Verification items for the finished model (mm, model axes). A direction names the side the tool comes from. Coordinates: 2 decimals unless noted, no trailing zeros. Order: outer loops, then holes, each group sorted by start corner. A loop starts at its lowest first (then second) coordinate and runs counter-clockwise, first axis right, second up. Notation, with made-up numbers: M 52.25,89 L 111.25,89 A33 cw 111.25,126 Z; hole C 77.5,-36.5 d1. An arc over 180 degrees is marked long. Answer as a JSON object with one key per item and string values. Group by question number.
(1) Cross-section at B-B (z = -0.7). Enter the section's corners in (x, y), plus the area to 3 significant figures.
(2) Gauge pin test, flat ends, axial feed: pin 1 Ø2 at (x, z) = (-15.5, -2.5) entering from -Y; pin 2 Ø2 at (x, z) = (-13.5, -1.5) entering from +Y; pin 3 Ø2 at (x, z) = (-7, -2.5) entering from +Y. Record the tip position at first contact, or that the pin passes through.
(3) Material ranges on line 1 (X direction, y = 3.5, z = -1.8); line 2 (X direction, y = 0.25, z = -0.95); line 3 (Y direction, x = -18.5, z = -1.65), recorded low to high.
(4) Cross-section at C-C (y = 3). Enter the section's corners in (x, z).
(5) Access from +Z, -Z, +X, -X, +Y, -Y to the whole of each face (thin tool, end or side, straight path). Record for faces 1 (the face through (-15, 3, 0)), 2 (the face through (-21.4, 5.48, -2.03)), 3 (the face through (-8.51, -0.51, -2.03)).
(6) Cross-section at A-A (x = -27.5). Enter the section's corners in (y, z).
(7) Cross-section at D-D (x = -10.5). Enter the section's corners in (y, z), plus the area to 3 significant figures.
from build123d import *

# Parameters (mm, degrees)
EXTRUDE_1_DEPTH = 4
FILLET_1_R      = 10


with BuildPart() as part:
    # ｽｹｯﾁ1 → ﾎﾞｽ - 押し出し1 (new body)
    with BuildSketch(Plane.XY):
        with BuildLine():
            Line((-0.345934077, 5), (0, 5))
            Line((0, 5), (0, 4.654065923))
            ThreePointArc((0, 4.654065923), (0.59354166, 3.648912529), (0.8, 2.5))
            ThreePointArc((0.8, 2.5), (0.59354166, 1.351087471), (0, 0.345934077))
            Line((0, 0.345934077), (0, 0))
            Line((0, 0), (-0.345934077, 0))
            ThreePointArc((-0.345934077, 0), (-2.5, -0.8), (-4.654065923, 0))
            Line((-4.654065923, 0), (-7.398979486, 0))
            ThreePointArc((-7.398979486, 0), (-1.214384811, -2.847634392), (3, 2.5))
            ThreePointArc((3, 2.5), (-1.214384811, 7.847634392), (-7.398979486, 5))
            Line((-7.398979486, 5), (-4.654065923, 5))
            ThreePointArc((-4.654065923, 5), (-2.5, 5.8), (-0.345934077, 5))
        make_face()
        with BuildLine():
            ThreePointArc((-4.654065923, 0), (-5.8, 2.5), (-4.654065923, 5))
            Line((-4.654065923, 5), (-7.398979486, 5))
            ThreePointArc((-7.398979486, 5), (-8, 2.5), (-7.398979486, 0))
            Line((-7.398979486, 0), (-4.654065923, 0))
        make_face()
        with BuildLine():
            Line((0, 0), (0, 0.345934077))
            ThreePointArc((0, 0.345934077), (-0.166547622, 0.166547622), (-0.345934077, 0))
            Line((-0.345934077, 0), (0, 0))
        make_face()
        with BuildLine():
            Line((0, 4.654065923), (0, 5))
            Line((0, 5), (-0.345934077, 5))
            ThreePointArc((-0.345934077, 5), (-0.166547622, 4.833452378), (0, 4.654065923))
        make_face()
        with BuildLine():
            ThreePointArc((-7.398979486, 0), (-8, 2.5), (-7.398979486, 5))
            Line((-7.398979486, 5), (-22.601020514, 5))
            ThreePointArc((-22.601020514, 5), (-22.152365608, 3.785615189), (-22, 2.5))
            ThreePointArc((-22, 2.5), (-22.152365608, 1.214384811), (-22.601020514, 0))
            Line((-22.601020514, 0), (-7.398979486, 0))
        make_face()
        with BuildLine():
            ThreePointArc((-22, 2.5), (-22.152365608, 3.785615189), (-22.601020514, 5))
            Line((-22.601020514, 5), (-25.345934077, 5))
            ThreePointArc((-25.345934077, 5), (-24.500131874, 3.875060445), (-24.2, 2.5))
            ThreePointArc((-24.2, 2.5), (-24.500131874, 1.124939555), (-25.345934077, 0))
            Line((-25.345934077, 0), (-22.601020514, 0))
            ThreePointArc((-22.601020514, 0), (-22.152365608, 1.214384811), (-22, 2.5))
        make_face()
        with BuildLine():
            Line((-25.345934077, 5), (-22.601020514, 5))
            ThreePointArc((-22.601020514, 5), (-33, 2.5), (-22.601020514, 0))
            Line((-22.601020514, 0), (-25.345934077, 0))
            ThreePointArc((-25.345934077, 0), (-27.5, -0.8), (-29.654065923, 0))
            Line((-29.654065923, 0), (-30, 0))
            Line((-30, 0), (-30, 0.345934077))
            ThreePointArc((-30, 0.345934077), (-30.8, 2.5), (-30, 4.654065923))
            Line((-30, 4.654065923), (-30, 5))
            Line((-30, 5), (-29.654065923, 5))
            ThreePointArc((-29.654065923, 5), (-27.5, 5.8), (-25.345934077, 5))
        make_face()
        with BuildLine():
            ThreePointArc((-30, 4.654065923), (-29.833452378, 4.833452378), (-29.654065923, 5))
            Line((-29.654065923, 5), (-30, 5))
            Line((-30, 5), (-30, 4.654065923))
        make_face()
        with BuildLine():
            Line((-30, 0), (-29.654065923, 0))
            ThreePointArc((-29.654065923, 0), (-29.833452378, 0.166547622), (-30, 0.345934077))
            Line((-30, 0.345934077), (-30, 0))
        make_face()
    extrude(amount=-EXTRUDE_1_DEPTH)

    # ﾌｨﾚｯﾄ1
    fillet_1_edges = [part.edges().sort_by_distance(p)[0] for p in [
        (-7.398979486, 0, -2),
        (-22.601020514, 0, -2),
        (-22.601020514, 5, -2),
        (-7.398979486, 5, -2),
    ]]
    fillet(fillet_1_edges, radius=FILLET_1_R)


solid = part.part
Taken from the geometry:
{
 "1": {"outline": "M -24.25,-1.94 A10 cw -18.33,0 L -11.67,0 A10 cw -5.75,-1.94 A5.5 ccw long -5.75,6.94 A10 cw -11.67,5 L -18.33,5 A10 cw -24.25,6.94 A5.5 ccw long Z; hole C -27.5,2.5 d6.6; hole C -2.5,2.5 d6.6", "area": "201 mm²"},
 "2": {"pin 1": "stops at y = 0", "pin 2": "stops at y = 5", "pin 3": "stops at y = 6.76"},
 "3": {"line 1": "x = -32.91 to -30.64, -24.36 to -5.64, 0.64 to 2.91", "line 2": "x = -32.52 to -29.91, -25.09 to -4.91, -0.09 to 2.52", "line 3": "y = 0 to 5"},
 "4": {"outline": "M -32.98,-4 L -30.76,-4 L -30.76,0 L -32.98,0 Z; M -24.24,-4 L -5.76,-4 L -5.76,0 L -24.24,0 Z; M 0.76,-4 L 2.98,-4 L 2.98,0 L 0.76,0 Z"},
 "5": {"face 1": "+Z, +X, -X, +Y, -Y", "face 2": "+Z, -Z, +Y", "face 3": "+Z, -Z, -Y"},
 "6": {"outline": "M -3,-4 L -0.8,-4 L -0.8,0 L -3,0 Z; M 5.8,-4 L 8,-4 L 8,0 L 5.8,0 Z"},
 "7": {"outline": "M -0.07,-4 L 5.07,-4 L 5.07,0 L -0.07,0 Z", "area": "20.5 mm²"}
}
